Source: three-view drawing plus pictorial views. Frame: mm from the lowest corner of the part. Give positions to 0.01 mm unless a question says otherwise; leave off trailing zeros. Loops run counter-clockwise (first coordinate to the right, second up) from the corner with the lowest first, then second, coordinate; pieces in that order, holes last.
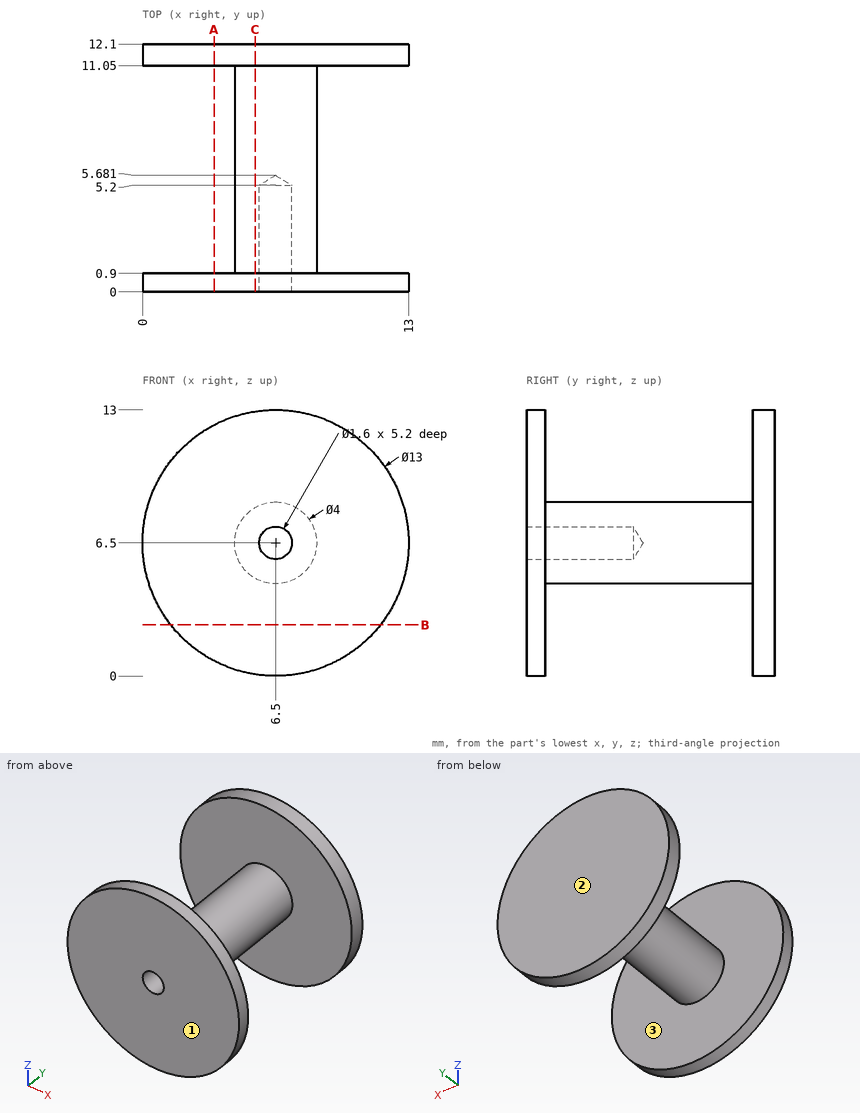
(1) Cut plane B-B (z = 2.5). Return the cut outline in (x, y), and give its area (3 significant figures).
Values follow:
outline: (1.38, 0) - (11.62, 0) - (11.62, 0.9) - (1.38, 0.9) - close; (1.38, 11.05) - (11.62, 11.05) - (11.62, 12.1) - (1.38, 12.1) - close
area: 20.0 mm2
(2) Ray query, probe 1 along X at (y, z) = (2.75, 6.5); probe 2 along Y at (x, z) = (6, 2.25); probe 3 along X at (y, z) = (11.5, 12) (1 decimal). Return the intervals inside material, ascending.
Values follow:
probe 1: x = 4.5 to 5.7, 7.3 to 8.5
probe 2: y = 0 to 0.9, 11.05 to 12.1
probe 3: x = 3 to 10
(3) Pin query (flat end, axial travel): pin 1 Ø4 at (x, z) = (9.5, 3.5) entering from -Y; pin 2 Ø5 at (x, y) = (6.5, 4.5) entering from +Z; pin 3 Ø3 at (x, y) = (10.5, 1.5) entering from +Z. Return the tip coordinate at first contact, or that it passes through.
Values follow:
pin 1: stops at y = 0
pin 2: stops at z = 8.5
pin 3: stops at z = 12.45
(4) Cut plane C-C (x = 5.5). Return the cut outline in (y, z).
Values follow:
outline: (0, 0.08) - (0.9, 0.08) - (0.9, 4.77) - (11.05, 4.77) - (11.05, 0.08) - (12.1, 0.08) - (12.1, 12.92) - (11.05, 12.92) - (11.05, 8.23) - (0.9, 8.23) - (0.9, 12.92) - (0, 12.92) - close
(5) Cut plane A-A (x = 3.5). Return the cut outline in (y, z), and give its area (3 significant figures).
Values follow:
outline: (0, 0.73) - (0.9, 0.73) - (0.9, 12.27) - (0, 12.27) - close; (11.05, 0.73) - (12.1, 0.73) - (12.1, 12.27) - (11.05, 12.27) - close
area: 22.5 mm2
(6) Mould query, pull axis Y, two halves, no side actions, for the marked faces 1, 2 and 3. Classes: +Y half, -Y half, draft (parallel to the pull), parting line (faces both ways), or undercut.
Values follow:
face 1: -Y half
face 2: +Y half
face 3: undercut
